CAD build for the part. Positions are in the model's coordinates, mm. A direction names the side the tool comes from. Give positions to 0.01 mm unless a question says otherwise; leave off trailing zeros. Order: outer loops, then holes, each group sorted by start corner. A loop starts at its lowest first (then second) coordinate and runs counter-clockwise, first axis right, second up. Notation, with made-up numbers: M 18.25,-16.75 L 74.25,-16.75 A20 cw 74.25,0.25 Z; hole C 59.25,7.5 d7. An arc over 180 degrees is marked long. Put each result on its own line as item: value. Start each with the question number.
1) Drill centre lines: line 1 (Y direction, x = 64.5, z = -2); line 2 (Z direction, x = 67.5, y = -20.2); line 3 (X direction, y = -20.75, z = 0). Where is each one in solid material? Low to high. Write a range as [from, to].
2) Tool access for faces 1 (the face through (66.6, 15.89, -0.04)), 2 (the face through (70, 21.75, 0)), 3 (the face through (67, -19.75, 0)), 4 (the face through (43, 19.25, 0)): list every direction of +Z, -Z, +X, -X, +Y, -Y with a clear straight run to the whole face (end or side of a thin tool).
3) Cut at A-A (x = 47). Write the cut outline in (y, z).
4) Two-plate mould, pull along X, no slides. Class faces 5 (the face through (53, 16.75, 0)), 6 (the face through (66, -21.75, 0)): released by +X, released by -X, zero draft, split by the parting line, or undercut.
5) Cut at D-D (z = -0.1). Give the number of separate pieces and of enclosed holes in the cut face, and give its area (3 significant figures).
6) Cut at B-B (y = 9.5). Write the cut outline in (x, z), and give its area (3 significant figures).
7) Cut at C-C (y = -5). Write the cut outline in (x, z).
8) Pin check, flat tips, straight feed: pin 1 (1.5 mm diameter, centred on x = 68.5, z = 0, fed in from -Y); pin 2 (2.5 mm diameter, centred on x = -67.5, z = 0, fed in from -Y); pin 3 (1.5 mm diameter, centred on x = -7.5, z = -0.5, fed in from +Y); pin 4 (1.5 mm diameter, centred on x = 67.5, z = 0, fed in from -Y). Stop position of each tip, or through.
Autodesk Inventor part; units mm, degrees
ref_plane "YZ Plane" through (0, 0, 0) normal (1, 0, 0) x (0, 1, 0)
ref_plane "XZ Plane" through (0, 0, 0) normal (0, 1, 0) x (-1, 0, 0)
ref_plane "XY Plane" through (0, 0, 0) normal (0, 0, 1) x (1, 0, 0)
sketch "スケッチ1" plane through (0, 0, 0) normal (0, 0, 1) x (1, 0, 0)
  line L0 (-72.5, -21.75) -> (72.5, -21.75) construction
  line L1 (72.5, -21.75) -> (72.5, 21.75) construction
  line L2 (72.5, 21.75) -> (-72.5, 21.75) construction
  line L3 (-72.5, 21.75) -> (-72.5, -21.75) construction
  line L4 (-72.5, -21.75) -> (72.5, 21.75) construction
  line L5 (72.5, -21.75) -> (-72.5, 21.75) construction
  line L6 (-67.5, 21.75) -> (-67.5, -21.75) construction
  line L7 (0, 0) -> (0, 21.75) construction
  line L8 (0, 0) -> (-72.5, 0) construction
  line L9 (67.5, 21.75) -> (67.5, -21.75) construction
  line L10 (-72.5, -21.75) -> (-61.6, -21.75)
  line L11 (49.5, 21.75) -> (49.5, 23.75)
  line L12 (49.5, 23.75) -> (62.5, 23.75)
  line L13 (62.5, 23.75) -> (62.5, 21.75)
  line L14 (66.6, 21.75) -> (72.5, 21.75)
  line L15 (72.5, 21.75) -> (72.5, -21.75)
  line L16 (72.5, -21.75) -> (61.6, -21.75)
  line L17 (-57.5, -21.75) -> (-57.5, -23.75)
  line L18 (-57.5, -23.75) -> (57.5, -23.75)
  line L19 (57.5, -23.75) -> (57.5, -21.75)
  arc A0 (45.4, 21.75) -> (49.5, 21.75) centre (47.45, 21.75) ccw
  arc A1 (62.5, 21.75) -> (66.6, 21.75) centre (64.55, 21.75) ccw
  arc A2 (-57.5, -21.75) -> (-61.6, -21.75) centre (-59.55, -21.75) ccw
  arc A3 (61.6, -21.75) -> (57.5, -21.75) centre (59.55, -21.75) ccw
  line L20 (-72.5, -21.75) -> (-72.5, -16.75)
  line L21 (-72.5, -16.75) -> (39.5, 21.75)
  line L22 (45.4, 21.75) -> (39.5, 21.75)
  line L23 (66.95, 24.476) -> (70.05, 24.476) construction
  line L24 (70.05, 24.476) -> (70.05, 13.3235) construction
  line L25 (70.05, 13.3235) -> (66.95, 13.3235) construction
  line L26 (66.95, 13.3235) -> (66.95, 24.476) construction
  line L27 (68.5, 24.476) -> (68.5, 13.3235) construction
  line L28 (41.95, 24.476) -> (45.05, 24.476) construction
  line L29 (45.05, 24.476) -> (45.05, 13.9945) construction
  line L30 (45.05, 13.9945) -> (41.95, 13.9945) construction
  line L31 (41.95, 13.9945) -> (41.95, 24.476) construction
  line L32 (43.5, 24.476) -> (43.5, 13.9945) construction
  dimension "d16" = 5
  dimension "d20" = 43.5
  dimension "d40" = 135
  dimension "d41" = 10
  dimension "d42" = 2.05
  dimension "d43" = 2
  dimension "d44" = 5
  dimension "d45" = 10
  dimension "d46" = 10
  dimension "d48" = 3.1
  dimension "d50" = 4
  dimension "d51" = 25
  dimension "d52" = 3.1
  dimension "d62" = 6
  dimension "d63" = 6
extrude "押し出し1" add sketch "スケッチ1" along normal blind 2.5
mirror "ミラー1" about plane through (8.4049, -6.8572, 0) normal (0, 0, -1) of "押し出し1"
sketch "スケッチ2" plane through (-72.5, -21.75, 2.5) normal (0, -1, 0) x (1, 0, 0)
  line L0 (0, -5) -> (0, 0)
  line L1 (15, -5) -> (130, -5) construction
  line L2 (72.5, -5) -> (72.5, 0) construction
  line L3 (15, 0) -> (130, 0) construction
  point P0 (72.5, -2.5)
  point P1 (140, -2.5)
  point P2 (0, -2.5)
hole "穴1" at (67.5, -21.75, 0) direction (0, 1, 0) diameter 2.459 depth 2
sketch "スケッチ4" plane through (66.6, 21.75, 2.5) normal (0, 1, 0) x (1, 0, 0)
  line L0 (5.9, 5) -> (5.9, 0)
  point P0 (-66.6, 2.5)
  point P1 (1.9, 2.5)
  point P2 (-23.1, 2.5)
  point P3 (5.9, 2.5)
  dimension "d53" = 4
  dimension "d54" = 25
hole "穴2" at (68.5, 21.75, 0) at (43.5, 21.75, 0) direction (0, -1, 0) diameter 2.459 depth 2.5
sketch "スケッチ6" plane through (0, 0, 2.5) normal (0, 0, 1) x (1, 0, 0)
  line L0 (61.6, -21.75) -> (72.5, -21.75)
  line L1 (72.5, -21.75) -> (72.5, 21.75)
  line L2 (72.5, 21.75) -> (66.6, 21.75)
  line L3 (39.5, 21.75) -> (-72.5, -16.75)
  line L4 (67.5, 16.75) -> (67.5, -16.75) construction
  line L5 (67.5, -16.75) -> (-57.1192, -16.75) construction
  line L6 (-57.1192, -16.75) -> (40.3354, 16.75) construction
  line L7 (40.3354, 16.75) -> (67.5, 16.75) construction
  line L8 (67.5, -16.75) -> (-8.3919, 0) construction
  line L9 (67.5, -14.1898) -> (67.5, 16.75)
  line L10 (67.5, 16.75) -> (40.3354, 16.75)
  line L11 (40.3354, 16.75) -> (-3.8563, 1.5591)
  line L12 (-3.8563, 1.5591) -> (67.5, -14.1898)
  line L13 (55.9002, -16.75) -> (-57.1192, -16.75)
  line L14 (-57.1192, -16.75) -> (-12.9275, -1.5591)
  line L15 (-12.9275, -1.5591) -> (55.9002, -16.75)
  point P0 (0, 0)
  dimension "d72" = 5
  dimension "d73" = 5
  dimension "d74" = 5
  dimension "d75" = 5
  dimension "d76" = 5
extrude "押し出し4" cut sketch "スケッチ6" against normal blind 10
fillet "フィレット3" radius 3 7 edges at (-3.8563, 1.5591, 0) (40.3354, 16.75, 0) (67.5, -14.1898, 0) (55.9002, -16.75, 0) (-12.9275, -1.5591, 0) (-57.1192, -16.75, 0) (67.5, 16.75, 0)
sketch "スケッチ7" plane through (-72.5, -21.75, 2.5) normal (0, -1, 0) x (1, 0, 0)
  line L0 (0, 0) -> (0, -5)
  line L1 (15, 0) -> (130, 0)
  line L2 (15, -5) -> (130, -5)
  line L3 (0, -2.5) -> (5, -2.5)
  point P0 (72.5, -2.5)
  dimension "d80" = 5
hole "穴3" at (-67.5, -21.75, 0) direction (0, 1, 0) diameter 3 end through all
equation "\"d16\" = d4"
equation "\"d40\" = d6"
equation "\"d41\" = d3"
equation "\"d46\" = d45"
equation "\"d63\" = d62"
equation "\"d73\" = d72"
equation "\"d74\" = d73"
equation "\"d75\" = d74"
equation "\"d76\" = d74"
properties part number "ForeArm_vertical_frame01" material "アセタール樹脂、黒"
Solution:
1. line 1: [-21.75, -13.46], [16.75, 19.7]
1. line 2: [-2.5, -1.23], [1.23, 2.5]
1. line 3: [-72.5, -69], [-66, -61.34], [-57.76, 57.76], [61.34, 66.27], [68.73, 72.5]
2. face 1: +Z, -Z
2. face 2: +Z, -Z, +X, +Y
2. face 3: -Y
2. face 4: +Y
3. outline: M -23.75,-2.5 L -9.67,-2.5 L -9.67,2.5 L -23.75,2.5 Z; M 16.75,-2.5 L 19.75,-2.5 L 19.75,2.5 L 16.75,2.5 Z
4. face 5: undercut
4. face 6: zero draft
5. separate pieces: 2
5. enclosed holes: 2
5. area: 2,310 mm²
6. outline: M 3.86,-2.5 L 19.24,-2.5 L 19.24,2.5 L 3.86,2.5 Z; M 67.5,-2.5 L 72.5,-2.5 L 72.5,2.5 L 67.5,2.5 Z
6. area: 102 mm²
7. outline: M -38.32,-2.5 L -22.94,-2.5 L -22.94,2.5 L -38.32,2.5 Z; M 2.66,-2.5 L 25.86,-2.5 L 25.86,2.5 L 2.66,2.5 Z; M 67.5,-2.5 L 72.5,-2.5 L 72.5,2.5 L 67.5,2.5 Z
8. pin 1: y = -21.75
8. pin 2: through
8. pin 3: y = 5.85
8. pin 4: y = -19.75
